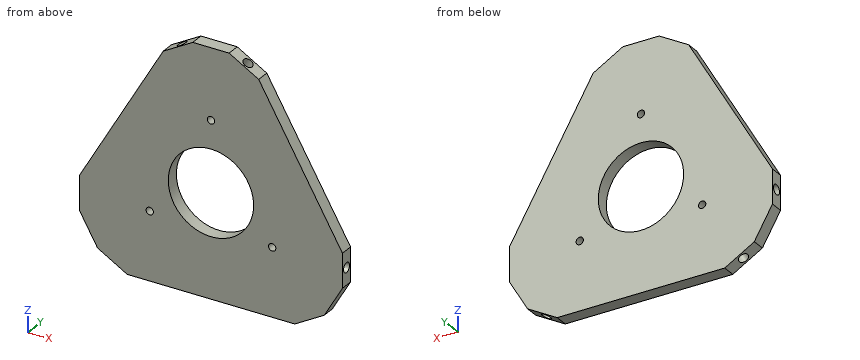
from build123d import *

# Parameters (mm, degrees)
BOSS_EXTRUDE2_DEPTH       = 5.4
F_3_0MM_DOWEL_HOLE1_D     = 4
F_3_0MM_DOWEL_HOLE1_DEPTH = 10
F_3_0MM_DOWEL_HOLE1_TIP   = 1.201721238
F_3_0MM_DOWEL_HOLE2_D     = 4
F_3_0MM_DOWEL_HOLE2_DEPTH = 10
F_3_0MM_DOWEL_HOLE2_TIP   = 1.201721238
F_3_0MM_DOWEL_HOLE3_D     = 4
F_3_0MM_DOWEL_HOLE3_DEPTH = 10
F_3_0MM_DOWEL_HOLE3_TIP   = 1.201721238
F_3_0MM_DOWEL_HOLE4_D     = 4
F_3_0MM_DOWEL_HOLE4_DEPTH = 10
F_3_0MM_DOWEL_HOLE4_TIP   = 1.201721238
F_3_0MM_DOWEL_HOLE5_D     = 4
F_3_0MM_DOWEL_HOLE5_DEPTH = 10
F_3_0MM_DOWEL_HOLE5_TIP   = 1.201721238
F_3_0MM_DOWEL_HOLE6_D     = 4
F_3_0MM_DOWEL_HOLE6_DEPTH = 10
F_3_0MM_DOWEL_HOLE6_TIP   = 1.201721238
SKETCH23_R                = 17.5
CUT_EXTRUDE1_DEPTH        = 211.795738776
CUT_EXTRUDE2_DEPTH        = 211.795738776
CUT_EXTRUDE2_DEPTH_BACK   = 211.795738776
SKETCH24_R                = 1.5


with BuildPart() as part:
    # Sketch1 → Boss-Extrude2 (new body)
    with BuildSketch(Plane(origin=(0, 0, 0), x_dir=(1, 0, 0), z_dir=(0, 1, 0))):
        Polygon((-181.608413742, -39.986262339), (-139.182006871, -113.470954622), (-108.123721459, -113.470954622), (-65.697314588, -39.986262339), (-81.226457294, -13.088998174), (-166.079271036, -13.088998174), align=None)
    extrude(amount=BOSS_EXTRUDE2_DEPTH)

    # Chamfer3
    # the kernel refuses this chamfer: 14 mm, written as the material it takes off along each edge
    with BuildSketch(Plane(origin=(-139.182006871, -21.431130006, 113.470954622), x_dir=(-0.5280200004833012, 0, -0.8492319348032166), z_dir=(0, 1, 0))) as chamfer3_piece_1:
        with BuildLine():
            Line((8.572452002, 0), (-4.761795885, -7.128270007))
            Line((-4.761795885, -7.128270007), (-4.999580826, -6.980424406))
            ThreePointArc((-4.999580826, -6.980424406), (-2.499790413, -3.490212203), (-0.237784942, 0.1478456))
            Line((-0.237784942, 0.1478456), (0.009145575, 0.2798506))
            ThreePointArc((0.009145575, 0.2798506), (4.290798789, 0.1399253), (8.581597577, 0.2798506))
            Line((8.581597577, 0.2798506), (8.572452002, 0))
        make_face()
    extrude(amount=48.262260012, mode=Mode.SUBTRACT)

    # Chamfer4
    # the kernel refuses this chamfer: 14 mm, written as the material it takes off along each edge
    with BuildSketch(Plane(origin=(-108.123721459, -21.431130006, 113.470954622), x_dir=(0.5280200004833001, 0, -0.8492319348032171), z_dir=(0, 1, 0))) as chamfer4_piece_1:
        with BuildLine():
            Line((8.572452002, 0), (-4.761795885, 7.128270007))
            Line((-4.761795885, 7.128270007), (-4.999580826, 6.980424406))
            ThreePointArc((-4.999580826, 6.980424406), (-2.499790413, 3.490212203), (-0.237784942, -0.1478456))
            Line((-0.237784942, -0.1478456), (0.009145575, -0.2798506))
            ThreePointArc((0.009145575, -0.2798506), (4.290798789, -0.1399253), (8.581597577, -0.2798506))
            Line((8.581597577, -0.2798506), (8.572452002, 0))
        make_face()
    extrude(amount=48.262260012, mode=Mode.SUBTRACT)

    # Chamfer5
    # the kernel refuses this chamfer: 14 mm, written as the material it takes off along each edge
    with BuildSketch(Plane(origin=(-65.697314588, -21.431130006, 39.986262339), x_dir=(-0.47144642900294653, 0, -0.8818947015264179), z_dir=(0, 1, 0))) as chamfer5_piece_1:
        with BuildLine():
            Line((8.572452002, 0), (-4.761795885, 7.128270007))
            Line((-4.761795885, 7.128270007), (-4.999580826, 6.980424406))
            ThreePointArc((-4.999580826, 6.980424406), (-2.499790413, 3.490212203), (-0.237784942, -0.1478456))
            Line((-0.237784942, -0.1478456), (0.009145575, -0.2798506))
            ThreePointArc((0.009145575, -0.2798506), (4.290798789, -0.1399253), (8.581597577, -0.2798506))
            Line((8.581597577, -0.2798506), (8.572452002, 0))
        make_face()
    extrude(amount=48.262260012, mode=Mode.SUBTRACT)

    # Chamfer6
    # the kernel refuses this chamfer: 14 mm, written as the material it takes off along each edge
    with BuildSketch(Plane(origin=(-81.226457294, -21.431130006, 13.088998174), x_dir=(0.5280200004833007, 0, 0.8492319348032168), z_dir=(0, 1, 0))) as chamfer6_piece_1:
        with BuildLine():
            Line((8.572452002, 0), (-4.761795885, -7.128270007))
            Line((-4.761795885, -7.128270007), (-4.999580826, -6.980424406))
            ThreePointArc((-4.999580826, -6.980424406), (-2.499790413, -3.490212203), (-0.237784942, 0.1478456))
            Line((-0.237784942, 0.1478456), (0.009145575, 0.2798506))
            ThreePointArc((0.009145575, 0.2798506), (4.290798789, 0.1399253), (8.581597577, 0.2798506))
            Line((8.581597577, 0.2798506), (8.572452002, 0))
        make_face()
    extrude(amount=48.262260012, mode=Mode.SUBTRACT)

    # Chamfer7
    # the kernel refuses this chamfer: 14 mm, written as the material it takes off along each edge
    with BuildSketch(Plane(origin=(-166.079271036, -21.431130006, 13.088998174), x_dir=(-0.5280200004833, 0, 0.8492319348032173), z_dir=(0, 1, 0))) as chamfer7_piece_1:
        with BuildLine():
            Line((8.572452002, 0), (-4.761795885, 7.128270007))
            Line((-4.761795885, 7.128270007), (-4.999580826, 6.980424406))
            ThreePointArc((-4.999580826, 6.980424406), (-2.499790413, 3.490212203), (-0.237784942, -0.1478456))
            Line((-0.237784942, -0.1478456), (0.009145575, -0.2798506))
            ThreePointArc((0.009145575, -0.2798506), (4.290798789, -0.1399253), (8.581597577, -0.2798506))
            Line((8.581597577, -0.2798506), (8.572452002, 0))
        make_face()
    extrude(amount=48.262260012, mode=Mode.SUBTRACT)

    # Chamfer8
    # the kernel refuses this chamfer: 14 mm, written as the material it takes off along each edge
    with BuildSketch(Plane(origin=(-181.608413742, -21.431130006, 39.986262339), x_dir=(0.4714464290029468, 0, 0.8818947015264177), z_dir=(0, 1, 0))) as chamfer8_piece_1:
        with BuildLine():
            Line((8.572452002, 0), (-4.761795885, 7.128270007))
            Line((-4.761795885, 7.128270007), (-4.999580826, 6.980424406))
            ThreePointArc((-4.999580826, 6.980424406), (-2.499790413, 3.490212203), (-0.237784942, -0.1478456))
            Line((-0.237784942, -0.1478456), (0.009145575, -0.2798506))
            ThreePointArc((0.009145575, -0.2798506), (4.290798789, -0.1399253), (8.581597577, -0.2798506))
            Line((8.581597577, -0.2798506), (8.572452002, 0))
        make_face()
    extrude(amount=48.262260012, mode=Mode.SUBTRACT)

    # Ø3.0mm Dowel Hole1
    with Locations(Plane(origin=(-81.909140423, 0, 141.870792817), x_dir=(0.8660254037844395, 0, 0.49999999999999856), z_dir=(-0.49999999999999856, 0, 0.8660254037844395))):
        with Locations((-63.799676389, 2.7)):
            Hole(F_3_0MM_DOWEL_HOLE1_D / 2, depth=F_3_0MM_DOWEL_HOLE1_DEPTH)
            with Locations((0, 0, -(F_3_0MM_DOWEL_HOLE1_DEPTH + F_3_0MM_DOWEL_HOLE1_TIP / 2))):  # 118° drill point
                Cone(0, F_3_0MM_DOWEL_HOLE1_D / 2, F_3_0MM_DOWEL_HOLE1_TIP, mode=Mode.SUBTRACT)

    # Ø3.0mm Dowel Hole2
    with Locations(Plane(origin=(20.08270834, 0, 34.784271199), x_dir=(0.8660254037844377, 0, -0.5000000000000018), z_dir=(0.5000000000000018, 0, 0.8660254037844377))):
        with Locations((-150.373366846, 2.7)):
            Hole(F_3_0MM_DOWEL_HOLE2_D / 2, depth=F_3_0MM_DOWEL_HOLE2_DEPTH)
            with Locations((0, 0, -(F_3_0MM_DOWEL_HOLE2_DEPTH + F_3_0MM_DOWEL_HOLE2_TIP / 2))):  # 118° drill point
                Cone(0, F_3_0MM_DOWEL_HOLE2_D / 2, F_3_0MM_DOWEL_HOLE2_TIP, mode=Mode.SUBTRACT)

    # Ø3.0mm Dowel Hole3
    with Locations(Plane(origin=(-69.738766472, 0, 0), x_dir=(0, 0, -1), z_dir=(1, 0, 0))):
        with Locations((-39.986262339, 2.7)):
            Hole(F_3_0MM_DOWEL_HOLE3_D / 2, depth=F_3_0MM_DOWEL_HOLE3_DEPTH)
            with Locations((0, 0, -(F_3_0MM_DOWEL_HOLE3_DEPTH + F_3_0MM_DOWEL_HOLE3_TIP / 2))):  # 118° drill point
                Cone(0, F_3_0MM_DOWEL_HOLE3_D / 2, F_3_0MM_DOWEL_HOLE3_TIP, mode=Mode.SUBTRACT)

    # Ø3.0mm Dowel Hole4
    with Locations(Plane(origin=(-27.99504273, 0, 48.488836368), x_dir=(-0.8660254037844382, 0, -0.5000000000000009), z_dir=(0.5000000000000009, 0, -0.8660254037844382))):
        with Locations((63.799676389, 2.7)):
            Hole(F_3_0MM_DOWEL_HOLE4_D / 2, depth=F_3_0MM_DOWEL_HOLE4_DEPTH)
            with Locations((0, 0, -(F_3_0MM_DOWEL_HOLE4_DEPTH + F_3_0MM_DOWEL_HOLE4_TIP / 2))):  # 118° drill point
                Cone(0, F_3_0MM_DOWEL_HOLE4_D / 2, F_3_0MM_DOWEL_HOLE4_TIP, mode=Mode.SUBTRACT)

    # Ø3.0mm Dowel Hole5
    with Locations(Plane(origin=(-33.831389353, 0, -58.597685249), x_dir=(-0.8660254037844384, 0, 0.5000000000000004), z_dir=(-0.5000000000000004, 0, -0.8660254037844384))):
        with Locations((150.373366846, 2.7)):
            Hole(F_3_0MM_DOWEL_HOLE5_D / 2, depth=F_3_0MM_DOWEL_HOLE5_DEPTH)
            with Locations((0, 0, -(F_3_0MM_DOWEL_HOLE5_DEPTH + F_3_0MM_DOWEL_HOLE5_TIP / 2))):  # 118° drill point
                Cone(0, F_3_0MM_DOWEL_HOLE5_D / 2, F_3_0MM_DOWEL_HOLE5_TIP, mode=Mode.SUBTRACT)

    # Ø3.0mm Dowel Hole6
    with Locations(Plane.ZY.offset(177.566961858)):
        with Locations((39.986262339, 2.7)):
            Hole(F_3_0MM_DOWEL_HOLE6_D / 2, depth=F_3_0MM_DOWEL_HOLE6_DEPTH)
            with Locations((0, 0, -(F_3_0MM_DOWEL_HOLE6_DEPTH + F_3_0MM_DOWEL_HOLE6_TIP / 2))):  # 118° drill point
                Cone(0, F_3_0MM_DOWEL_HOLE6_D / 2, F_3_0MM_DOWEL_HOLE6_TIP, mode=Mode.SUBTRACT)

    # Sketch23 → Cut-Extrude1 (cut, through all)
    with BuildSketch(Plane(origin=(0, 5.4, 0), x_dir=(1, 0, 0), z_dir=(0, 1, 0))):
        with Locations(Location((-123.652864165, -55.515405045, 0), (0, 0, 270))):
            Circle(SKETCH23_R)
    extrude(amount=-CUT_EXTRUDE1_DEPTH, mode=Mode.SUBTRACT)

    # Sketch24 → Cut-Extrude2 (cut, two sides: drawn at the far end of the back side and taken through both)
    with BuildSketch(Plane(origin=(0, 5.4, 0), x_dir=(1, 0, 0), z_dir=(0, 1, 0)).offset(-CUT_EXTRUDE2_DEPTH_BACK)):
        with Locations(Location((-98.557375053, -41.02651765, 0), (0, 0, 270))):
            Circle(SKETCH24_R)
        with Locations(Location((-148.748353277, -41.02651765, 0), (0, 0, 270))):
            Circle(SKETCH24_R)
        with Locations(Location((-123.652864165, -84.493179833, 0), (0, 0, 270))):
            Circle(SKETCH24_R)
    extrude(amount=CUT_EXTRUDE2_DEPTH + CUT_EXTRUDE2_DEPTH_BACK, mode=Mode.SUBTRACT)


solid = part.part
CAD build for the part. Positions are in the model's coordinates, mm. Coordinates: 2 decimals unless noted, no trailing zeros. Write each loop counter-clockwise with the first axis right and the second up, starting at its lowest first coordinate (ties: lowest second). Pieces come first, ordered by that corner, then holes. Notation, with made-up numbers: M 16.25,8.25 L 42.25,8.25 A17 ccw 42.25,14.25 Z; hole C 54,-12 d9. An arc over 180 degrees is marked long. Answer as a JSON object with one key per item and string values. Group by question number.
1) Saw through at A-A (z = 57.5). Write the cut outline in (x, y), plus the area to 3 significant figures.
2) Pin check, flat tips, straight feed: pin 1 Ø1.5 at (y, z) = (2.5, 97) entering from +X; pin 2 Ø1.5 at (x, y) = (-159, 3.5) entering from -Z; pin 3 Ø1.5 at (y, z) = (4.5, 83.5) entering from -X. Stop position of each tip, or through.
3) Saw through at C-C (y = 1.7). Give the number of separate pieces and of enclosed holes in the cut face, plus the area to 3 significant figures.
4) Saw through at D-D (z = 80.5). Write the cut outline in (x, y), plus the area to 3 significant figures.
5) Wall check: line 1 (Y direction, x = -137, z = 109); line 2 (X direction, y = 1.7, z = 45.5); line 3 (Z direction, x = -172.25, y = 2.7). Give the ranges that are in metal, low to high. Write a range as from..to.
6) Saw through at B-B (x = -154). Write the cut outline in (y, z), plus the area to 3 significant figures.
Values follow:
{
 "1": {"outline": "M -171.5,0 L -141.04,0 L -141.04,5.4 L -171.5,5.4 Z; M -106.27,0 L -75.81,0 L -75.81,5.4 L -106.27,5.4 Z", "area": "329 mm2"},
 "2": {"pin 1": "stops at x = -98.18", "pin 2": "stops at z = 13.24", "pin 3": "stops at x = -156.92"},
 "3": {"separate pieces": "1", "enclosed holes": "4", "area": "6,730 mm2"},
 "4": {"outline": "M -158.22,0 L -89.09,0 L -89.09,5.4 L -158.22,5.4 Z", "area": "373 mm2"},
 "5": {"line 1": "y = 0..0.73, 4.67..5.4", "line 2": "x = -177.57..-138, -109.3..-69.74", "line 3": "z = 23.78..37.99, 41.99..56.2"},
 "6": {"outline": "M 0,13.09 L 5.4,13.09 L 5.4,87.81 L 0,87.81 Z", "area": "403 mm2"}
}
